```python
from build123d import *

# Parameters (mm, degrees)
F0_W     = 112.086874
F0_H     = 36.914836
F1_DEPTH = 3


with BuildPart() as f1:
    # F0 (on Top) → F1 (new body)
    with BuildSketch(Plane.XY):
        Rectangle(F0_W, F0_H)
        Polygon((-40.794464, 9.361871), (-29.940543, 9.437671), (-24.447938, 0.0758), (-29.809254, -9.361871), (-40.663174, -9.437671), (-46.155779, -0.0758), align=None, mode=Mode.SUBTRACT)
        Polygon((8.495988, 0), (3.040028, -9.45), (-7.871892, -9.45), (-13.327852, 0), (-7.871892, 9.45), (3.040028, 9.45), align=None, mode=Mode.SUBTRACT)
        Polygon((42.875068, 0), (37.39024, -9.5), (26.420585, -9.5), (20.935758, 0), (26.420585, 9.5), (37.39024, 9.5), align=None, mode=Mode.SUBTRACT)
    extrude(amount=F1_DEPTH)


solid = f1.part
```
Read the model definition and answer for the solid it produces. Units are mm, in the model's axes. A direction names the side the tool comes from. Give positions to 0.01 mm unless a question says otherwise; leave off trailing zeros. Write each loop counter-clockwise with the first axis right and the second up, starting at its lowest first coordinate (ties: lowest second). Pieces come first, ordered by that corner, then holes. Notation, with made-up numbers: (-5, 26) -> (39, 26) arc R11 cw to (39, 31) -> close; hole circle Ø3 at (4.25, 53). An arc over 180 degrees is marked (long way). Answer in a Markdown table with one row per item.
1) Section A-A on x = -0.5 is taken. Give the vertices of the cut face in (y, z), plus the area to 3 significant figures.
Results list:
| item | result |
|---|---|
| outline | (-18.46, 0) -> (-9.45, 0) -> (-9.45, 3) -> (-18.46, 3) -> close; (9.45, 0) -> (18.46, 0) -> (18.46, 3) -> (9.45, 3) -> close |
| area | 54.0 mm^2 |
2) Determine the mould class of faces 3 (the flat face through (23.64, 4.68, 1.48)), 4 (the flat face through (-1, 18.457, 1)), 5 (the flat face through (56.043, 0, 1)) for opening direction X: released by +X, released by -X, zero draft, split by the parting line, or undercut.
Results list:
| item | result |
|---|---|
| face 3 | undercut |
| face 4 | zero draft |
| face 5 | released by +X |
3) A tool of negligible diameter and unlimited length cuts with its end or side. For faces 1 (the flat face through (5.806, -4.659, 1.479)), 2 (the flat face through (-1, 13, 3)), from which of +Z, -Z, +X, -X, +Y, -Y can it reach the whole face along a straight path? Write none if from no direction.
Results list:
| item | result |
|---|---|
| face 1 | +Z, -Z |
| face 2 | +Z, +X, -X, +Y, -Y |
4) Section C-C on y = -6.5 is taken. Give the vertices of the cut face in (x, z).
Results list:
| item | result |
|---|---|
| outline | (-56.04, 0) -> (-42.39, 0) -> (-42.39, 3) -> (-56.04, 3) -> close; (-28.18, 0) -> (-9.58, 0) -> (-9.58, 3) -> (-28.18, 3) -> close; (4.74, 0) -> (24.69, 0) -> (24.69, 3) -> (4.74, 3) -> close; (39.12, 0) -> (56.04, 0) -> (56.04, 3) -> (39.12, 3) -> close |
5) Section D-D on x = -43 is taken. Give the vertices of the cut face in (y, z).
Results list:
| item | result |
|---|---|
| outline | (-18.46, 0) -> (-5.45, 0) -> (-5.45, 3) -> (-18.46, 3) -> close; (5.48, 0) -> (18.46, 0) -> (18.46, 3) -> (5.48, 3) -> close |
6) Section B-B on z = 1.8 is taken. Give the vertices of the cut face in (x, y).
Results list:
| item | result |
|---|---|
| outline | (-56.04, -18.46) -> (56.04, -18.46) -> (56.04, 18.46) -> (-56.04, 18.46) -> close; hole (-46.16, -0.08) -> (-40.66, -9.44) -> (-29.81, -9.36) -> (-24.45, 0.08) -> (-29.94, 9.44) -> (-40.79, 9.36) -> close; hole (-13.33, 0) -> (-7.87, -9.45) -> (3.04, -9.45) -> (8.5, 0) -> (3.04, 9.45) -> (-7.87, 9.45) -> close; hole (20.94, 0) -> (26.42, -9.5) -> (37.39, -9.5) -> (42.88, 0) -> (37.39, 9.5) -> (26.42, 9.5) -> close |
7) Straight lines are drawn through the part: line 1 (Y direction, x = 27.5, z = 1.5); line 2 (Y direction, x = -40, z = 1.15); line 3 (X direction, y = 4.5, z = 2.75). For each, find the intervals that lie inside material, in ascending order. Write a range as [from, to].
Results list:
| item | result |
|---|---|
| line 1 | [-18.46, -9.5], [9.5, 18.46] |
| line 2 | [-18.46, -9.43], [9.37, 18.46] |
| line 3 | [-56.04, -43.56], [-27.04, -10.73], [5.9, 23.53], [40.28, 56.04] |
